```python
from build123d import *

# Parameters (mm, degrees)
EXTRUDE_1_DEPTH = 660


with BuildPart() as part:
    # 草图5 → 凸台-拉伸1 (new body, symmetric)
    with BuildSketch(Plane(origin=(0, 0, 0), x_dir=(1, 0, 0), z_dir=(0, 1, 0))):
        with BuildLine():
            Line((190, 0), (190, -23.210187215))
            Line((190, -23.210187215), (11.76, -58.836233734))
            ThreePointArc((11.76, -58.836233734), (0, -60), (-11.76, -58.836233734))
            Line((-11.76, -58.836233734), (-190, -23.210187215))
            Line((-190, -23.210187215), (-190, 0))
            Line((-190, 0), (-190, 23.210187215))
            Line((-190, 23.210187215), (-11.759999967, 58.836233741))
            ThreePointArc((-11.759999967, 58.836233741), (1.7e-08, 60), (11.76, 58.836233734))
            Line((11.76, 58.836233734), (190, 23.210187215))
            Line((190, 23.210187215), (190, 0))
        make_face()
    extrude(amount=EXTRUDE_1_DEPTH, both=True)


solid = part.part
```
Read the model definition and answer for the solid it produces. Units are mm, in the model's axes. Give positions to 0.01 mm unless a question says otherwise; leave off trailing zeros. Write each loop counter-clockwise with the first axis right and the second up, starting at its lowest first coordinate (ties: lowest second). Pieces come first, ordered by that corner, then holes. Notation, with made-up numbers: (71.5, 74.25) - (83.5, 74.25) arc R6 cw to (83.5, 78.25) - close; hole circle Ø3 at (55, -21.5). An arc over 180 degrees is marked (long way). Write item = value, one per line. Start each with the question number.
Item 1: Find section A-A (y = 366.5). Give the vertices of the cut face in (x, z).
Item 2: Find section C-C (z = -44.5). Give the vertices of the cut face in (x, y), then the cut area to 3 significant figures.
Item 3: Find section B-B (x = -107). Give the vertices of the cut face in (y, z).
Item 4: Each of these flat-tipped pins is pushed along its axis until it touches: P1, Ø3, axis at x = -137.5, y = -118, coming from the +Z side; P2, Ø12, axis at x = 53.5, y = 52.5, coming from the -Z side; P3, Ø5, axis at x = 115.5, z = -41, coming from the +Y side. Where does it stop, or does it pass through?
Item 5: Find the intervals of material crossed by probe 1 along Z at (x, y) = (0.5, -334.5); probe 2 along Z at (x, y) = (-38.5, -484), in increasing order. Write a range as [from, to].
Response:
q1.outline = (-190, -23.21) - (-11.76, -58.84) arc R60 ccw to (11.76, -58.84) - (190, -23.21) - (190, 23.21) - (11.76, 58.84) arc R60 ccw to (-11.76, 58.84) - (-190, 23.21) - close
q2.outline = (-83.49, -660) - (83.49, -660) - (83.49, 660) - (-83.49, 660) - close
q2.area = 220,000 mm²
q3.outline = (-660, -39.8) - (660, -39.8) - (660, 39.8) - (-660, 39.8) - close
q4.P1 = 34
q4.P2 = -51.69
q4.P3 = through
q5.probe_1 = [-60, 60]
q5.probe_2 = [-53.49, 53.49]
